```python
from build123d import *

# Parameters (mm, degrees)
F0_R     = 1.016
F0_R_2   = 46.355
F1_DEPTH = 5.08
F3_DEPTH = 25.4


with BuildPart() as f1:
    # F0 (on Front) → F1 (new body)
    with BuildSketch(Plane.XZ):
        with BuildLine():
            Line((217.7707480356, 125.73), (72.5902493452, 125.73))
            Line((72.5902493452, 125.73), (25.4, 125.73))
            Line((25.4, 125.73), (25.4, 120.396))
            Line((25.4, 120.396), (-25.4, 120.396))
            Line((-25.4, 120.396), (-25.4, 125.73))
            Line((-25.4, 125.73), (-57.9255525078, 125.73))
            ThreePointArc((-57.9255525078, 125.73), (-70.6255525078, 122.3270452561), (-79.9225977639, 113.03))
            Line((-79.9225977639, 113.03), (-96.1853740178, 84.8620452561))
            Line((-96.1853740178, 84.8620452561), (-91.565994514, 82.1950452561))
            Line((-91.565994514, 82.1950452561), (-116.965994514, 38.2009547439))
            Line((-116.965994514, 38.2009547439), (-121.5853740178, 40.8679547439))
            Line((-121.5853740178, 40.8679547439), (-137.8481502717, 12.7))
            ThreePointArc((-137.8481502717, 12.7), (-141.2511050156, 0), (-137.8481502717, -12.7))
            Line((-137.8481502717, -12.7), (-121.5853740178, -40.8679547439))
            Line((-121.5853740178, -40.8679547439), (-116.965994514, -38.2009547439))
            Line((-116.965994514, -38.2009547439), (-91.565994514, -82.1950452561))
            Line((-91.565994514, -82.1950452561), (-96.1853740178, -84.8620452561))
            Line((-96.1853740178, -84.8620452561), (-79.9225977639, -113.03))
            ThreePointArc((-79.9225977639, -113.03), (-70.6255525078, -122.3270452561), (-57.9255525078, -125.73))
            Line((-57.9255525078, -125.73), (-25.4, -125.73))
            Line((-25.4, -125.73), (-25.4, -120.396))
            Line((-25.4, -120.396), (25.4, -120.396))
            Line((25.4, -120.396), (25.4, -125.73))
            Line((25.4, -125.73), (72.5902493452, -125.73))
            Line((72.5902493452, -125.73), (217.7707480356, -125.73))
            Line((217.7707480356, -125.73), (264.9609973808, -125.73))
            Line((264.9609973808, -125.73), (264.9609973808, -120.396))
            Line((264.9609973808, -120.396), (315.7609973808, -120.396))
            Line((315.7609973808, -120.396), (315.7609973808, -125.73))
            Line((315.7609973808, -125.73), (348.2865498886, -125.73))
            ThreePointArc((348.2865498886, -125.73), (360.9865498886, -122.3270452561), (370.2835951448, -113.03))
            Line((370.2835951448, -113.03), (386.5463713987, -84.8620452561))
            Line((386.5463713987, -84.8620452561), (381.9269918949, -82.1950452561))
            Line((381.9269918949, -82.1950452561), (407.3269918949, -38.2009547439))
            Line((407.3269918949, -38.2009547439), (411.9463713987, -40.8679547439))
            Line((411.9463713987, -40.8679547439), (428.2091476526, -12.7))
            ThreePointArc((428.2091476526, -12.7), (431.6121023964, 0), (428.2091476526, 12.7))
            Line((428.2091476526, 12.7), (411.9463713987, 40.8679547439))
            Line((411.9463713987, 40.8679547439), (407.3269918949, 38.2009547439))
            Line((407.3269918949, 38.2009547439), (381.9269918949, 82.1950452561))
            Line((381.9269918949, 82.1950452561), (386.5463713987, 84.8620452561))
            Line((386.5463713987, 84.8620452561), (370.2835951448, 113.03))
            ThreePointArc((370.2835951448, 113.03), (360.9865498886, 122.3270452561), (348.2865498886, 125.73))
            Line((348.2865498886, 125.73), (315.7609973808, 125.73))
            Line((315.7609973808, 125.73), (315.7609973808, 120.396))
            Line((315.7609973808, 120.396), (264.9609973808, 120.396))
            Line((264.9609973808, 120.396), (264.9609973808, 125.73))
            Line((264.9609973808, 125.73), (217.7707480356, 125.73))
        make_face()
        with Locations((87.2430986904, -87.63)):
            Circle(F0_R, mode=Mode.SUBTRACT)
        with Locations((-31.75, -57.15)):
            Circle(F0_R, mode=Mode.SUBTRACT)
        with Locations((-80.2159486953, -30.2848859509)):
            Circle(F0_R, mode=Mode.SUBTRACT)
        with Locations((16.7159486953, -30.2848859509)):
            Circle(F0_R, mode=Mode.SUBTRACT)
        with Locations((203.1178986904, -87.63)):
            Circle(F0_R, mode=Mode.SUBTRACT)
        with Locations((273.6450486855, -30.2848859509)):
            Circle(F0_R, mode=Mode.SUBTRACT)
        with Locations((322.1109973808, -57.15)):
            Circle(F0_R, mode=Mode.SUBTRACT)
        with Locations((370.5769460762, -30.2848859509)):
            Circle(F0_R, mode=Mode.SUBTRACT)
        with Locations((-80.2159486953, 30.2848859509)):
            Circle(F0_R, mode=Mode.SUBTRACT)
        with Locations((-31.75, 0)):
            Circle(F0_R_2, mode=Mode.SUBTRACT)
        with Locations((-31.75, 57.15)):
            Circle(F0_R, mode=Mode.SUBTRACT)
        with Locations((16.7159486953, 30.2848859509)):
            Circle(F0_R, mode=Mode.SUBTRACT)
        with Locations((87.2430986904, 87.63)):
            Circle(F0_R, mode=Mode.SUBTRACT)
        with Locations((273.6450486855, 30.2848859509)):
            Circle(F0_R, mode=Mode.SUBTRACT)
        with Locations((322.1109973808, 0)):
            Circle(F0_R_2, mode=Mode.SUBTRACT)
        with Locations((370.5769460762, 30.2848859509)):
            Circle(F0_R, mode=Mode.SUBTRACT)
        with Locations((322.1109973808, 57.15)):
            Circle(F0_R, mode=Mode.SUBTRACT)
        with Locations((203.1178986904, 87.63)):
            Circle(F0_R, mode=Mode.SUBTRACT)
    extrude(amount=F1_DEPTH)

    # F2 (on face) → F3 (join)
    with BuildSketch(Plane.XZ.offset(5.08)):
        with BuildLine():
            Line((74.056719029, 128.27), (-59.3920221915, 128.27))
            ThreePointArc((-59.3920221915, 128.27), (-72.0920221915, 124.8670452561), (-81.3890674477, 115.57))
            Line((-81.3890674477, 115.57), (-140.7810896392, 12.7))
            ThreePointArc((-140.7810896392, 12.7), (-144.1840443831, 0), (-140.7810896392, -12.7))
            Line((-140.7810896392, -12.7), (-81.3890674477, -115.57))
            ThreePointArc((-81.3890674477, -115.57), (-72.0920221915, -124.8670452561), (-59.3920221915, -128.27))
            Line((-59.3920221915, -128.27), (74.056719029, -128.27))
            Line((74.056719029, -128.27), (349.3600802049, -128.27))
            ThreePointArc((349.3600802049, -128.27), (362.0600802049, -124.8670452561), (371.357125461, -115.57))
            Line((371.357125461, -115.57), (430.7491476526, -12.7))
            ThreePointArc((430.7491476526, -12.7), (434.1521023964, 0), (430.7491476526, 12.7))
            Line((430.7491476526, 12.7), (371.357125461, 115.57))
            ThreePointArc((371.357125461, 115.57), (362.0600802049, 124.8670452561), (349.3600802049, 128.27))
            Line((349.3600802049, 128.27), (215.9113389844, 128.27))
            Line((215.9113389844, 128.27), (74.056719029, 128.27))
        make_face()
        with BuildLine():
            Line((-57.9255525078, 125.73), (-25.4, 125.73))
            Line((-25.4, 125.73), (25.4, 125.73))
            Line((25.4, 125.73), (264.9609973808, 125.73))
            Line((264.9609973808, 125.73), (315.7609973808, 125.73))
            Line((315.7609973808, 125.73), (348.2865498886, 125.73))
            ThreePointArc((348.2865498886, 125.73), (360.9865498886, 122.3270452561), (370.2835951448, 113.03))
            Line((370.2835951448, 113.03), (386.5463713987, 84.8620452561))
            Line((386.5463713987, 84.8620452561), (411.9463713987, 40.8679547439))
            Line((411.9463713987, 40.8679547439), (428.2091476526, 12.7))
            ThreePointArc((428.2091476526, 12.7), (431.6121023964, 0), (428.2091476526, -12.7))
            Line((428.2091476526, -12.7), (411.9463713987, -40.8679547439))
            Line((411.9463713987, -40.8679547439), (386.5463713987, -84.8620452561))
            Line((386.5463713987, -84.8620452561), (370.2835951448, -113.03))
            ThreePointArc((370.2835951448, -113.03), (360.9865498886, -122.3270452561), (348.2865498886, -125.73))
            Line((348.2865498886, -125.73), (315.7609973808, -125.73))
            Line((315.7609973808, -125.73), (264.9609973808, -125.73))
            Line((264.9609973808, -125.73), (25.4, -125.73))
            Line((25.4, -125.73), (-25.4, -125.73))
            Line((-25.4, -125.73), (-57.9255525078, -125.73))
            ThreePointArc((-57.9255525078, -125.73), (-70.6255525078, -122.3270452561), (-79.9225977639, -113.03))
            Line((-79.9225977639, -113.03), (-96.1853740178, -84.8620452561))
            Line((-96.1853740178, -84.8620452561), (-121.5853740178, -40.8679547439))
            Line((-121.5853740178, -40.8679547439), (-137.8481502717, -12.7))
            ThreePointArc((-137.8481502717, -12.7), (-141.2511050156, 0), (-137.8481502717, 12.7))
            Line((-137.8481502717, 12.7), (-121.5853740178, 40.8679547439))
            Line((-121.5853740178, 40.8679547439), (-96.1853740178, 84.8620452561))
            Line((-96.1853740178, 84.8620452561), (-79.9225977639, 113.03))
            ThreePointArc((-79.9225977639, 113.03), (-70.6255525078, 122.3270452561), (-57.9255525078, 125.73))
        make_face(mode=Mode.SUBTRACT)
    extrude(amount=-F3_DEPTH)


solid = f1.part
```
Check sheet for the modelled part. Datum: model origin and axes. Units: mm. A direction names the side the tool comes from. Coordinates: 2 decimals unless noted, no trailing zeros. Order: outer loops, then holes, each group sorted by start corner. A loop starts at its lowest first (then second) coordinate and runs counter-clockwise, first axis right, second up. Notation, with made-up numbers: M 14,-15 L 18,-15 A15 ccw 18,6 Z; hole C 83,-30 d8. An arc over 180 degrees is marked long. One line per question, with ' | ' between items. Start each with the question number.
Item 1: Access from +Z, -Z, +X, -X, +Y, -Y to the whole of each face (thin tool, end or side, straight path). Record for faces 4 (the flat face through (142, 7, -128.27)), 5 (the cylindrical face through (-141.25, 10.02, -0.19)), 6 (the flat face through (394.449, -2.504, -60.506)).
Item 2: Mould release check, pull along X, two halves, no side actions. Record for faces 1 (the flat face through (-108.48, 7.44, -63.57)), 2 (the cylindrical face through (-71.93, 7.44, 124.96)), 3 (the flat face through (400.637, 7.442, -64.855)): pulls with the +X half, pulls with the -X half, needs draft (parallel to the pull), parting line crosses it, or undercut.
Item 3: Sectioned sample at C-C on x = 336. Record the cut outline in (y, z).
Item 4: Gauge pin test, flat ends, axial feed: P1, Ø2, axis at y = 0, z = 30.5, coming from the +X side; P2, Ø3.5, axis at x = 370.58, z = 30.28, coming from the +Y side; P3, Ø1.5, axis at y = 6.5, z = 68.5, coming from the -X side. Record the tip position at first contact, or that the pin passes through.
Item 5: Material ranges on line 1 (Z direction, x = 62, y = 16); line 2 (X direction, y = -3.35, z = 87.63); line 3 (Y direction, x = 1.5, z = -95), recorded low to high.
Item 6: Sectioned sample at A-A on y = 12.25. Record the cut outline in (x, z).
Item 7: Sectioned sample at D-D on x = 162. Record the cut outline in (y, z), and give its area (3 significant figures).
Item 8: Sectioned sample at B-B on z = 0. Record the cut outline in (x, y) (3 decimals), and give its area (3 significant figures).
Answer below:
1) face 4: -Z, +X, -X, +Y, -Y | face 5: +Y | face 6: +Y, -Y
2) face 1: undercut | face 2: pulls with the -X half | face 3: pulls with the +X half
3) outline: M -5.08,-128.27 L 20.32,-128.27 L 20.32,-125.73 L 0,-125.73 L 0,-44.23 L -5.08,-44.23 Z; M -5.08,44.23 L 0,44.23 L 0,125.73 L 20.32,125.73 L 20.32,128.27 L -5.08,128.27 Z
4) P1: stops at x = 421.05 | P2: stops at y = 0 | P3: stops at x = -109
5) line 1: z = -128.27 to -125.73, 125.73 to 128.27 | line 2: x = -97.52 to 86.23, 88.26 to 202.1, 204.13 to 387.49 | line 3: y = -5.08 to 0
6) outline: M -140.78,-12.7 L -81.39,-115.57 A25.4 ccw -59.39,-128.27 L 349.36,-128.27 A25.4 ccw 371.36,-115.57 L 430.75,-12.7 A25.4 ccw 430.75,12.7 L 371.36,115.57 A25.4 ccw 349.36,128.27 L -59.39,128.27 A25.4 ccw -81.39,115.57 L -140.78,12.7 A25.4 ccw Z; hole M -137.85,-12.7 L -79.92,-113.03 A25.4 ccw -57.93,-125.73 L 348.29,-125.73 A25.4 ccw 370.28,-113.03 L 428.21,-12.7 A25.4 ccw 428.21,12.7 L 370.28,113.03 A25.4 ccw 348.29,125.73 L -57.93,125.73 A25.4 ccw -79.92,113.03 L -137.85,12.7 A25.4 ccw Z
7) outline: M -5.08,-128.27 L 20.32,-128.27 L 20.32,-125.73 L 0,-125.73 L 0,125.73 L 20.32,125.73 L 20.32,128.27 L -5.08,128.27 Z | area: 1,410 mm^2
8) outline: M -144.184,-5.08 L -78.105,-5.08 L -78.105,0 L -141.251,0 L -141.251,20.32 L -144.184,20.32 Z; M 14.605,-5.08 L 275.756,-5.08 L 275.756,0 L 14.605,0 Z; M 368.466,-5.08 L 434.152,-5.08 L 434.152,20.32 L 431.612,20.32 L 431.612,0 L 368.466,0 Z | area: 2,110 mm^2
